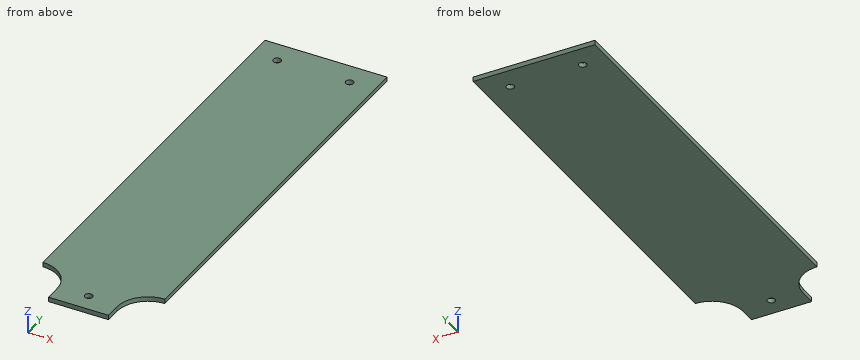
```python
from build123d import *

# Parameters (mm, degrees)
ESQUISSE1_R      = 2.5
EXTRUSION1_DEPTH = 3


with BuildPart() as part:
    # Esquisse1 → Extrusion1 (new body)
    with BuildSketch(Plane.XY):
        with BuildLine():
            Line((39.5, 292), (-39.5, 292))
            Line((-39.5, 292), (-39.5, 30))
            ThreePointArc((-39.5, 30), (-25.357864376, 24.142135624), (-19.5, 10))
            Line((-19.5, 10), (-19.5, 0))
            Line((-19.5, 0), (19.5, 0))
            Line((19.5, 0), (19.5, 10))
            ThreePointArc((19.5, 10), (25.357864376, 24.142135624), (39.5, 30))
            Line((39.5, 30), (39.5, 292))
        make_face()
        with Locations((-23.5, 277)):
            Circle(ESQUISSE1_R, mode=Mode.SUBTRACT)
        with Locations((23.5, 277)):
            Circle(ESQUISSE1_R, mode=Mode.SUBTRACT)
        with Locations((0, 12)):
            Circle(ESQUISSE1_R, mode=Mode.SUBTRACT)
    extrude(amount=EXTRUSION1_DEPTH)


solid = part.part
```
Read the model definition and answer for the solid it produces. Units are mm, in the model's axes. Give positions to 0.01 mm unless a question says otherwise; leave off trailing zeros. Order: outer loops, then holes, each group sorted by start corner. A loop starts at its lowest first (then second) coordinate and runs counter-clockwise, first axis right, second up.
(1) Find section A-A (z = 2.2). Give the vertices of the cut face in (x, y), plus the area to 3 significant figures.
(2) Given pin 1 (0.9 mm diameter, centred on y = 4, z = 1.5, fed in from -X); pin 2 (3 mm diameter, centred on x = 0, y = 12, fed in from -Z), each flat-ended and moving along its own axis, determine where each tip first touches the part or whether it passes through.
(3) Straight lines are drawn through the part: L1, parallel to X at y = 277, z = 2; L2, parallel to Y at x = 0.5, z = 2.2; L3, parallel to Y at x = 0, z = 0.75. For each, find the intervals that lie inside material, in ascending order.
(4) Find section C-C (x = -23.5). Give the vertices of the cut face in (y, z), plus the area to 3 significant figures.
(5) Find section B-B (x = 0). Give the vertices of the cut face in (y, z), plus the area to 3 significant figures.
Result sheet:
1. outline: (-39.5, 30) arc R20 cw to (-19.5, 10) - (-19.5, 0) - (19.5, 0) - (19.5, 10) arc R20 cw to (39.5, 30) - (39.5, 292) - (-39.5, 292) - close; hole circle Ø5 at (-23.5, 277); hole circle Ø5 at (0, 12); hole circle Ø5 at (23.5, 277)
1. area: 22,000 mm2
2. pin 1: stops at x = -19.5
2. pin 2: passes through
3. L1: x = -39.5 to -26, -21 to 21, 26 to 39.5
3. L2: y = 0 to 9.55, 14.45 to 292
3. L3: y = 0 to 9.5, 14.5 to 292
4. outline: (22, 0) - (274.5, 0) - (274.5, 3) - (22, 3) - close; (279.5, 0) - (292, 0) - (292, 3) - (279.5, 3) - close
4. area: 795 mm2
5. outline: (0, 0) - (9.5, 0) - (9.5, 3) - (0, 3) - close; (14.5, 0) - (292, 0) - (292, 3) - (14.5, 3) - close
5. area: 861 mm2
